The listing builds one solid part. Answer for the finished solid, in the listing's coordinates (mm). A direction names the side the tool comes from. Give positions to 0.01 mm unless a question says otherwise; leave off trailing zeros. Order: outer loops, then holes, each group sorted by start corner. A loop starts at its lowest first (then second) coordinate and runs counter-clockwise, first axis right, second up. Notation, with made-up numbers: (-22.5, 10) -> (3.5, 10) arc R23 ccw to (3.5, 23) -> close; hole circle Ø1 at (-6.75, 61). An arc over 180 degrees is marked (long way). Answer as a JSON object with one key per item and string values. Group by question number.
```python
from build123d import *

# Parameters (mm, degrees)
F0_W     = 88.9
F0_H     = 762
F1_DEPTH = 44.45
F2_W     = 25.4
F2_H     = 101.6
F3_DEPTH = 127
F4_R     = 6.35
F5_DEPTH = 127


with BuildPart() as f1:
    # F0 (on Front) → F1 (new body, symmetric)
    with BuildSketch(Plane.XZ):
        with Locations((-1.4848271385, 327.3150383137)):
            Rectangle(F0_W, F0_H)
    extrude(amount=F1_DEPTH, both=True)

    # F2 (on Right) → F3 (cut, symmetric)
    with BuildSketch(Plane.YZ):
        with Locations((0, 657.5150383137)):
            Rectangle(F2_W, F2_H)
    extrude(amount=F3_DEPTH, both=True, mode=Mode.SUBTRACT)

    # F4 (on face) → F5 (cut, symmetric)
    with BuildSketch(Plane(origin=(0, 44.45, 0), x_dir=(-1, 0, 0), z_dir=(0, 1, 0))):
        with Locations((0, 663.8650383137)):
            Circle(F4_R)
    extrude(amount=F5_DEPTH, both=True, mode=Mode.SUBTRACT)


solid = f1.part
```
(1) Flat-ended cylindrical pins translate along their axes: pin 1 Ø10 at (x, z) = (0, 663.87) entering from +Y; pin 2 Ø8 at (x, y) = (12.5, -4.5) entering from +Z. Find the tip coordinate at first contact, or state that the pin passes through.
(2) A cutting plane is placed at C-C (y = -6). Determine the outline of the cut face in (x, z), and give its area (3 significant figures).
(3) Which of the six approach directions +Z, -Z, +X, -X, +Y, -Y give full straight-line access (tool end or side, diameter ignored) to faces 1 (the cylindrical face through (1.377, 28.797, 657.666)), 2 (the flat face through (-1, 0, 606.715))?
(4) A cutting plane is placed at B-B (x = 0). Determine the outline of the cut face in (y, z).
(5) For a pull along Y with two mould halves and no side action, classify faces 3 (the flat face through (-1, -12.7, 657)), 4 (the flat face through (-2, -44.45, 333)), 5 (the cylindrical face through (1.377, -28.353, 657.666)), 6 (the flat face through (-2, 44.45, 333)) as +Y half, -Y half, draft (parallel to the pull), parting line (faces both ways), or undercut.
(6) Find the intervals of material crossed by line 1 along Z through (x, y) = (0, -22.5); line 2 along Y through (x, z) = (-11, 654.5); line 3 along Z through (x, y) = (-6, 7.5), in increasing order. Write a range as [from, to].
(7) A cutting plane is placed at A-A (z = 629.5). Determine the outline of the cut face in (x, y), and give its area (3 significant figures).
Check sheet entries:
{
 "1": {"pin 1": "passes through", "pin 2": "stops at z = 606.72"},
 "2": {"outline": "(-45.93, -53.68) -> (42.97, -53.68) -> (42.97, 606.72) -> (-45.93, 606.72) -> close", "area": "58,700 mm2"},
 "3": {"face 1": "+Y, -Y", "face 2": "+Z, +X, -X"},
 "4": {"outline": "(-44.45, -53.68) -> (44.45, -53.68) -> (44.45, 657.52) -> (12.7, 657.52) -> (12.7, 606.72) -> (-12.7, 606.72) -> (-12.7, 657.52) -> (-44.45, 657.52) -> close; (-44.45, 670.22) -> (-12.7, 670.22) -> (-12.7, 708.32) -> (-44.45, 708.32) -> close; (12.7, 670.22) -> (44.45, 670.22) -> (44.45, 708.32) -> (12.7, 708.32) -> close"},
 "5": {"face 3": "undercut", "face 4": "-Y half", "face 5": "draft", "face 6": "+Y half"},
 "6": {"line 1": "z = [-53.68, 657.52], [670.22, 708.32]", "line 2": "y = [-44.45, -12.7], [12.7, 44.45]", "line 3": "z = [-53.68, 606.72]"},
 "7": {"outline": "(-45.93, -44.45) -> (42.97, -44.45) -> (42.97, -12.7) -> (-45.93, -12.7) -> close; (-45.93, 12.7) -> (42.97, 12.7) -> (42.97, 44.45) -> (-45.93, 44.45) -> close", "area": "5,650 mm2"}
}
